Autodesk Inventor part; units mm, degrees
ref_plane "YZ Plane" through (0, 0, 0) normal (1, 0, 0) x (0, 1, 0)
ref_plane "XZ Plane" through (0, 0, 0) normal (0, 1, 0) x (-1, 0, 0)
ref_plane "XY Plane" through (0, 0, 0) normal (0, 0, 1) x (1, 0, 0)
sketch "Sketch1" plane through (0, 0, 0) normal (1, 0, 0) x (0, 1, 0)
  line L0 (57.15, 31.75) -> (-57.15, 31.75)
  line L1 (-57.15, 31.75) -> (-57.15, -31.75)
  line L2 (-57.15, -31.75) -> (57.15, -31.75)
  line L3 (57.15, -31.75) -> (57.15, 31.75)
  line L4 (-50.8, 25.4) -> (50.8, 25.4)
  line L5 (50.8, 25.4) -> (50.8, -25.4)
  line L6 (50.8, -25.4) -> (-50.8, -25.4)
  line L7 (-50.8, -25.4) -> (-50.8, 25.4)
  point P0 (0, 0)
  point P1 (0, -31.75)
  point P2 (57.15, 0)
  point P3 (0, 25.4)
  point P4 (-50.8, 0)
  dimension "d0" = 63.5
  dimension "d1" = 114.3
  dimension "d14" = 50.8
  dimension "d15" = 101.6
extrude "Extrusion1" add sketch "Sketch1" along normal blind 12.7 contours L3 L2 L1 L0 | L4 L5 L6 L7
sketch "Sketch2" plane through (12.7, 0, 0) normal (1, 0, 0) x (0, 0, -1)
  line L0 (-10.795, -15.24) -> (10.795, 15.24) construction
  line L1 (-10.795, 15.24) -> (10.795, -15.24) construction
  circle A0 centre (0, 0) radius 6.5484
  dimension "d5" = 30.48
  dimension "d12" = 13.0969
  dimension "d13" = 21.59
sketch "Sketch3" plane through (0, 0, 0) normal (-1, 0, 0) x (0, 0, 1)
  line L0 (-28.575, -53.975) -> (28.575, -53.975)
  line L1 (28.575, -53.975) -> (28.575, 53.975)
  line L2 (28.575, 53.975) -> (-28.575, 53.975)
  line L3 (-28.575, 53.975) -> (-28.575, -53.975)
  line L4 (22.098, 47.498) -> (22.098, -47.498)
  line L5 (22.098, -47.498) -> (-22.098, -47.498)
  line L6 (-22.098, -47.498) -> (-22.098, 47.498)
  line L7 (-22.098, 47.498) -> (22.098, 47.498)
  point P0 (0, 0)
  point P1 (0, -53.975)
  point P2 (-28.575, 0)
  point P3 (0, 0)
  point P4 (28.575, 0)
  point P5 (0, 53.975)
  dimension "d16" = 107.95
  dimension "d17" = 57.15
  dimension "d31" = 6.477
extrude "Extrusion3" cut sketch "Sketch3" against normal blind 3.175
extrude "Extrusion4" cut sketch "Sketch2" against normal through all
hole "Hole1" at (12.7, -15.24, 10.795) at (12.7, 15.24, 10.795) at (12.7, 15.24, -10.795) at (12.7, -15.24, -10.795) direction (-1, 0, 0) diameter 2.159 depth 8.8646 tip angle 118
fillet "Fillet1" radius 3.175 8 edges at (1.5875, 53.975, 28.575) (1.5875, -47.498, 22.098) (1.5875, -47.498, -22.098) (1.5875, -53.975, -28.575) (1.5875, 47.498, -22.098) (1.5875, -53.975, 28.575) (1.5875, 53.975, -28.575) (1.5875, 47.498, 22.098)
properties part number "plate" material "Aluminum 6061"
Geometry: final body of the model. Coordinates: model frame, mm. A direction names the side the tool comes from. Coordinates: 2 decimals unless noted, no trailing zeros. Order: outer loops, then holes, each group sorted by start corner. A loop starts at its lowest first (then second) coordinate and runs counter-clockwise, first axis right, second up. Notation, with made-up numbers: M -22.5,-11 L -13.5,-11 A22 cw -13.5,12 Z; hole C 11,39.25 d5. An arc over 180 degrees is marked long. Answer in a Markdown table with one row per item. Add a question column.
Q1. Section query D-D on z = 8.5. Return the cut outline in (x, y) (3 decimals), and give its area (3 significant figures).
Q2. Reachability of faces 4 (the flat face through (2, 47.498, 0)), 5 (the flat face through (6, -1, -31.75)), 6 (the cylindrical face through (8.2, 16.2, 10.3)) from +Z, -Z, +X, -X, +Y, -Y: full face, straight path, thin tool, end or side. Return the list, or none.
Q3. Contact query for flat-ended pins moving along their axis: P1, Ø8, axis at y = 0, z = 0, coming from the -X side; P2, Ø1.7, axis at y = 15.24, z = 10.795, coming from the +X side. Output: stop coordinate, or through.
Q4. Section query A-A on z = 0. Return the cut outline in (x, y) (3 decimals), and give its area (3 significant figures).
Q5. Mould query, pull axis Y, two halves, no side actions, for faces 1 (the flat face through (6, -57.15, 0)), 2 (the flat face through (6, 57.15, 0)), 3 (the flat face through (2, -47.498, 0)). Classes: released by +Y, released by -Y, zero draft, split by the parting line, or undercut.
Q6. Line query: L1, parallel to Z at x = 0.75, y = 34 (3 decimals); L2, parallel to Y at x = 2.5, z = 0 (3 decimals); L3, parallel to Z at x = 6.25, y = -15.24. Output: solid intervals per line, ascending.
Q7. Section query C-C on y = 0. Return the cut outline in (x, z) (3 decimals), and give its area (3 significant figures).
Q8. Section query B-B on x = 6.75. Count the separate pieces of the cut face and the enclosed holes in it, and give its area (3 significant figures).
Completed:
| question | item | result |
|---|---|---|
| 1 | outline | M 0,-57.15 L 12.7,-57.15 L 12.7,57.15 L 0,57.15 L 0,53.975 L 3.175,53.975 L 3.175,47.498 L 0,47.498 L 0,-47.498 L 3.175,-47.498 L 3.175,-53.975 L 0,-53.975 Z |
| 1 | area | 1,410 mm2 |
| 2 | face 4 | -X |
| 2 | face 5 | -Z, +X, -X, +Y, -Y |
| 2 | face 6 | +X |
| 3 | P1 | passes through |
| 3 | P2 | stops at x = 3.7 |
| 4 | outline | M 0,-57.15 L 12.7,-57.15 L 12.7,-6.548 L 0,-6.548 L 0,-47.498 L 3.175,-47.498 L 3.175,-53.975 L 0,-53.975 Z; M 0,6.548 L 12.7,6.548 L 12.7,57.15 L 0,57.15 L 0,53.975 L 3.175,53.975 L 3.175,47.498 L 0,47.498 Z |
| 4 | area | 1,240 mm2 |
| 5 | face 1 | released by -Y |
| 5 | face 2 | released by +Y |
| 5 | face 3 | undercut |
| 6 | L1 | z = -31.75 to -28.575, -22.098 to 22.098, 28.575 to 31.75 |
| 6 | L2 | y = -57.15 to -53.975, -47.498 to -6.548, 6.548 to 47.498, 53.975 to 57.15 |
| 6 | L3 | z = -31.75 to -11.87, -9.72 to 9.72, 11.87 to 31.75 |
| 7 | outline | M 0,-31.75 L 12.7,-31.75 L 12.7,-6.548 L 0,-6.548 L 0,-22.098 L 3.175,-22.098 L 3.175,-28.575 L 0,-28.575 Z; M 0,6.548 L 12.7,6.548 L 12.7,31.75 L 0,31.75 L 0,28.575 L 3.175,28.575 L 3.175,22.098 L 0,22.098 Z |
| 7 | area | 599 mm2 |
| 8 | separate pieces | 1 |
| 8 | enclosed holes | 5 |
| 8 | area | 7,110 mm2 |
